Can you work these out from the model? Positions are in its coordinate system, mm. A direction names the side the tool comes from. Give positions to 0.01 mm unless a question says otherwise; leave off trailing zeros. Write each loop counter-clockwise with the first axis right and the second up, starting at its lowest first coordinate (ties: lowest second). Pieces come first, ordered by that corner, then holes.
Autodesk Inventor part; units mm, degrees
ref_plane "YZ Plane" through (0, 0, 0) normal (1, 0, 0) x (0, 1, 0)
ref_plane "XZ Plane" through (0, 0, 0) normal (0, 1, 0) x (-1, 0, 0)
ref_plane "XY Plane" through (0, 0, 0) normal (0, 0, 1) x (1, 0, 0)
sketch "Sketch1" plane through (0, 0, 0) normal (0, 1, 0) x (-1, 0, 0)
  line L0 (0, 6.665) -> (0, 4.1495) construction
  line L1 (0, 4.1495) -> (0, 0) construction
  line L2 (-1.665, 6.4537) -> (-1.665, 3.1237)
  line L3 (-1.665, 3.1237) -> (1.665, 3.1237)
  line L4 (1.665, 3.1237) -> (1.665, 6.4537)
  line L5 (1.665, 6.4537) -> (-1.665, 3.1237) construction
  line L6 (-1.665, 6.4537) -> (1.665, 3.1237) construction
  line L7 (-6.665, 0) -> (-4.1495, 0) construction
  line L8 (-4.1495, 0) -> (0, 0) construction
  line L9 (-6.4537, -1.665) -> (-3.1237, -1.665)
  line L10 (-3.1237, -1.665) -> (-3.1237, 1.665)
  line L11 (-3.1237, 1.665) -> (-6.4537, 1.665)
  line L12 (-6.4537, 1.665) -> (-3.1237, -1.665) construction
  line L13 (-6.4537, -1.665) -> (-3.1237, 1.665) construction
  line L14 (0, -6.665) -> (0, -4.1495) construction
  line L15 (0, -4.1495) -> (0, 0) construction
  line L16 (1.665, -6.4537) -> (1.665, -3.1237)
  line L17 (1.665, -3.1237) -> (-1.665, -3.1237)
  line L18 (-1.665, -3.1237) -> (-1.665, -6.4537)
  line L19 (-1.665, -6.4537) -> (1.665, -3.1237) construction
  line L20 (1.665, -6.4537) -> (-1.665, -3.1237) construction
  line L21 (6.665, 0) -> (4.1495, 0) construction
  line L22 (4.1495, 0) -> (0, 0) construction
  line L23 (6.4537, 1.665) -> (3.1237, 1.665)
  line L24 (3.1237, 1.665) -> (3.1237, -1.665)
  line L25 (3.1237, -1.665) -> (6.4537, -1.665)
  line L26 (6.4537, -1.665) -> (3.1237, 1.665) construction
  line L27 (6.4537, 1.665) -> (3.1237, -1.665) construction
  arc A0 (-1.665, 6.4537) -> (-6.4537, 1.665) centre (0, 0) ccw
  arc A1 (-6.4537, -1.665) -> (-1.665, -6.4537) centre (0, 0) ccw
  arc A2 (1.665, -6.4537) -> (6.4537, -1.665) centre (0, 0) ccw
  arc A3 (6.4537, 1.665) -> (1.665, 6.4537) centre (0, 0) ccw
  point P0 (0, 4.7887)
  point P1 (-4.7887, 0)
  point P2 (0, -4.7887)
  point P3 (4.7887, 0)
  dimension "d1" = 3.33
  dimension "d4" = 360
extrude "Extrusion1" add sketch "Sketch1" along normal blind 3.33
sketch "Sketch2" plane through (-1.665, 0, 6.4537) normal (1, 0, 0) x (0, 0, -1)
  line L0 (3.33, 0) -> (3.33, 3.33) construction
  line L1 (3.33, 1.665) -> (0, 1.665) construction
  line L2 (0, 0) -> (0, 3.33) construction
  circle A0 centre (1.665, 1.665) radius 1.33
  point P0 (6.4537, 0)
  dimension "d8" = 2.66
extrude "Extrusion2" add sketch "Sketch2" along normal blind 3.33
pattern_circular "Circular Pattern1" count 4 over 360 about axis through (0, 0, 0) along (0, 1, 0) of "Extrusion2"
sketch "Sketch3" plane through (0, 3.33, 0) normal (0, 1, 0) x (1, 0, 0)
  circle A0 centre (0, 0) radius 1
  dimension "d14" = 2
extrude "Extrusion3" add sketch "Sketch3" along normal blind 30
properties part number "G-6"
(1) For faces 1 (the face through (4.748, 1.642, 4.678)), 2 (the face through (-3.124, 2, 0)), 3 (the face through (-6.29, 1.64, 1.665)), which set-ups out of +Z, -Z, +X, -X, +Y, -Y let a thin tool reach every point of the face, with its end or its side?
Returned:
face 1: +Z, +X, +Y, -Y
face 2: +Y, -Y
face 3: none
(2) Will these pins go through, and if not, where does the flat tip stop? P1, Ø1, axis at y = 2, z = 0.5, coming from the +X side; P2, Ø2, axis at x = -1, y = 9.5, coming from the +Z side; P3, Ø2.5, axis at y = 2.5, z = -5.5, coming from the -X side.
Returned:
P1: stops at x = 6.12
P2: stops at z = 1
P3: stops at x = -5.13
(3) Imagine slicing it at A-A, the plane z = 0. Write out the boundary of the cut face in (x, y) (3 decimals).
Returned:
outline: circle Ø2.66 at (-4.789, 1.665); (-3.124, 0) - (3.124, 0) - (3.124, 3.33) - (1, 3.33) - (1, 33.33) - (-1, 33.33) - (-1, 3.33) - (-3.124, 3.33) - close; circle Ø2.66 at (4.789, 1.665)
(4) Imagine slicing it at C-C, the plane x = 5.5. Write out the boundary of the cut face in (y, z) (3 decimals), plus the area to 3 significant figures.
Returned:
outline: (0, -3.765) - (3.33, -3.765) - (3.33, -1.665) - (2.789, -1.665) - (2.789, 1.665) - (3.33, 1.665) - (3.33, 3.765) - (0, 3.765) - (0, 1.665) - (0.541, 1.665) - (0.541, -1.665) - (0, -1.665) - close
area: 21.5 mm2
(5) If I drill on L1, parallel to Y at x = 1, z = -2.5; L2, parallel to X at y = 3, z = -3.75 (3 decimals); L3, parallel to Z at x = 0, y = 31, over which ranges is the centre line in solid material (lowest first)?
Returned:
L1: y = 0 to 3.33
L2: x = -5.51 to -1.665, 1.665 to 5.51
L3: z = -1 to 1
(6) If we mould it in two halves opening along X, with no side actions, what happens to faces 4 (the face through (-4.678, 1.642, 4.748)), 5 (the face through (0, 2, -3.124)), 6 (the face through (0, 18, -1))? For each: +X half, -X half, draft (parallel to the pull), parting line (faces both ways), or undercut.
Returned:
face 4: -X half
face 5: undercut
face 6: parting line
(7) Imagine slicing it at D-D, the plane y = 9. Write out the boundary of the cut face in (x, z).
Returned:
outline: circle Ø2 at (0, 0)
(8) Imagine slicing it at B-B, the plane x = 0. Write out the boundary of the cut face in (y, z) (3 decimals), plus the area to 3 significant figures.
Returned:
outline: (0, -3.124) - (3.33, -3.124) - (3.33, -1) - (33.33, -1) - (33.33, 1) - (3.33, 1) - (3.33, 3.124) - (0, 3.124) - close; circle Ø2.66 at (1.665, -4.789); circle Ø2.66 at (1.665, 4.789)
area: 91.9 mm2
